```python
from build123d import *

# Parameters (mm, degrees)
BOSS_EXTRU_1_DEPTH      = 4
ESQUISSE2_R             = 1
ENL_V_MAT_EXTRU_1_DEPTH = 257.850637531
D_GAGEMENT_M31_D        = 3.4
D_GAGEMENT_M31_DEPTH    = 10
D_GAGEMENT_M31_TIP      = 1.021463052
CONG_1_R                = 5


with BuildPart() as part:
    # Esquisse1 → Boss.-Extru.1 (new body)
    with BuildSketch(Plane(origin=(0, 0, 0), x_dir=(1, 0, 0), z_dir=(0, 1, 0))):
        Polygon((-92.5, 0), (92.5, 0), (132.5, 40), (132.5, 220), (102.5, 220), (85.179491924, 190), (-85.179491924, 190), (-102.5, 220), (-132.5, 220), (-132.5, 40), align=None)
    extrude(amount=BOSS_EXTRU_1_DEPTH)

    # Esquisse2 → Enlèv. mat.-Extru.1 (cut, through all)
    with BuildSketch(Plane(origin=(0, 4, 0), x_dir=(1, 0, 0), z_dir=(0, 1, 0))):
        with Locations(Location((70, 8, 0), (0, 0, 270))):
            Circle(ESQUISSE2_R)
        with Locations(Location((124.5, 70, 0), (0, 0, 270))):
            Circle(ESQUISSE2_R)
        with Locations(Location((124.5, 212, 0), (0, 0, 270))):
            Circle(ESQUISSE2_R)
        with Locations(Location((-70, 8, 0), (0, 0, 90))):
            Circle(ESQUISSE2_R)
        with Locations(Location((-124.5, 70, 0), (0, 0, 90))):
            Circle(ESQUISSE2_R)
        with Locations(Location((-124.5, 212, 0), (0, 0, 90))):
            Circle(ESQUISSE2_R)
    extrude(amount=-ENL_V_MAT_EXTRU_1_DEPTH, mode=Mode.SUBTRACT)

    # Dégagement M31
    with Locations(Plane(origin=(0, 4, 0), x_dir=(1, 0, 0), z_dir=(0, 1, 0))):
        with Locations((-70, 8), (70, 8), (124.5, 70), (124.5, 212), (-124.5, 212), (-124.5, 70)):
            Hole(D_GAGEMENT_M31_D / 2, depth=D_GAGEMENT_M31_DEPTH)
            with Locations((0, 0, -(D_GAGEMENT_M31_DEPTH + D_GAGEMENT_M31_TIP / 2))):  # 118° drill point
                Cone(0, D_GAGEMENT_M31_D / 2, D_GAGEMENT_M31_TIP, mode=Mode.SUBTRACT)

    # Congé1
    cong_1_edges = [part.edges().sort_by_distance(p)[0] for p in [
        (132.5, 2, -220),
        (132.5, 2, -40),
        (92.5, 2, 0),
        (-92.5, 2, 0),
        (-132.5, 2, -40),
        (-132.5, 2, -220),
        (-102.5, 2, -220),
        (-85.179491924, 2, -190),
        (85.179491924, 2, -190),
        (102.5, 2, -220),
    ]]
    fillet(cong_1_edges, radius=CONG_1_R)


solid = part.part
```
CAD build for the part. Positions are in the model's coordinates, mm. Give positions to 0.01 mm unless a question says otherwise; leave off trailing zeros. Write each loop counter-clockwise with the first axis right and the second up, starting at its lowest first coordinate (ties: lowest second). Pieces come first, ordered by that corner, then holes. Notation, with made-up numbers: M -33.75,3 L 0.25,3 A23 ccw 0.25,25 Z; hole C -20.75,26.25 d2. An arc over 180 degrees is marked long. Return JSON: item names as keys, results as strings. Group by question number.
(1) Band-saw the part on B-B (x = 113.5). Give the cut face in (y, z).
(2) Drill centre lines: L1, parallel to X at y = 3.15, z = -70; L2, parallel to X at y = 2.8, z = -9; L3, parallel to X at y = 2.25, z = -212. Where is each one in solid material? Low to high. Write a range as [from, to].
(3) Flat gauge pin, fed straight in: pin 1 Ø12 at (x, z) = (-89.5, -83.5) entering from -Y. Where does the tip first touch, or does it go through?
(4) Band-saw the part on A-A (y = 1.15). Give the cut face in (x, z), and give its area (3 significant figures).
(5) Mould opens along X. For faces 1 (the face through (-2, 4, -112)), 2 (the face through (112.2, 2, -19.7)), 3 (the face through (93.941, 1.972, -205.175)), 4 (the face through (-93.739, 1.972, -204.825)) say: pulls with the +X half, pulls with the -X half, needs draft (parallel to the pull), parting line crosses it, or undercut.
(6) Band-saw the part on C-C (x = -116). Give the cut face in (y, z), and give its area (3 significant figures).
Entries:
{
 "1": {"outline": "M 0,-220 L 4,-220 L 4,-21 L 0,-21 Z"},
 "2": {"L1": "x = [-132.5, -126.2], [-122.8, 122.8], [126.2, 132.5]", "L2": "x = [-101.5, -71.37], [-68.63, 68.63], [71.37, 101.5]", "L3": "x = [-132.5, -126.2], [-122.8, -97.88], [97.88, 122.8], [126.2, 132.5]"},
 "3": {"pin 1": "stops at y = 0"},
 "4": {"outline": "M -132.5,-215 A5 ccw -127.5,-220 L -105.39,-220 A5 ccw -101.06,-217.5 L -86.62,-192.5 A5 cw -82.29,-190 L 82.29,-190 A5 cw 86.62,-192.5 L 101.06,-217.5 A5 ccw 105.39,-220 L 127.5,-220 A5 ccw 132.5,-215 L 132.5,-42.07 A5 ccw 131.04,-38.54 L 93.96,-1.46 A5 ccw 90.43,0 L -90.43,0 A5 ccw -93.96,-1.46 L -131.04,-38.54 A5 ccw -132.5,-42.07 Z; hole C -124.5,-212 d3.4; hole C -124.5,-70 d3.4; hole C -70,-8 d3.4; hole C 70,-8 d3.4; hole C 124.5,-212 d3.4; hole C 124.5,-70 d3.4", "area": "51,000 mm^2"},
 "5": {"face 1": "needs draft", "face 2": "pulls with the +X half", "face 3": "undercut", "face 4": "undercut"},
 "6": {"outline": "M 0,-220 L 4,-220 L 4,-23.5 L 0,-23.5 Z", "area": "786 mm^2"}
}
